Answer from the drawing. Dimensions are ordinates in mm from the lowest x, y and z of the part. A direction names the side the tool comes from. Coordinates: 2 decimals unless noted, no trailing zeros. Loops run counter-clockwise (first coordinate to the right, second up) from the corner with the lowest first, then second, coordinate; pieces in that order, holes last.
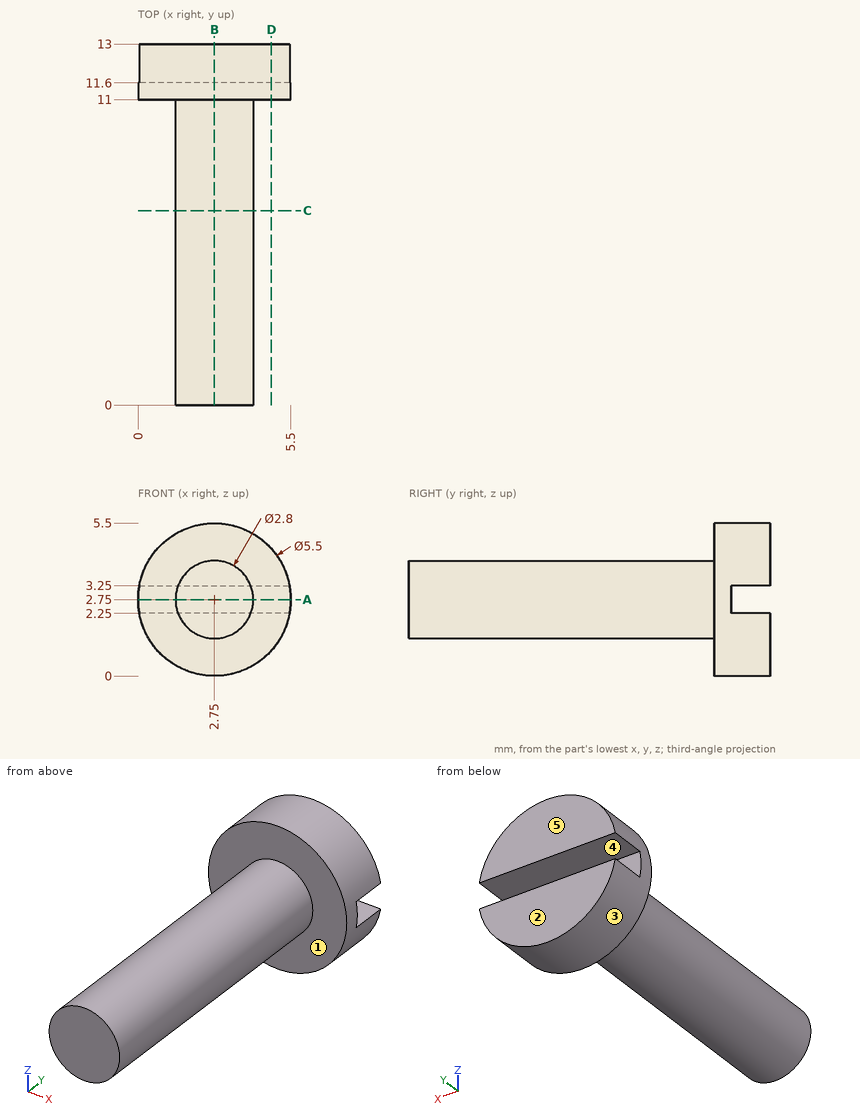
Item 1: A cutting plane is placed at B-B on x = 2.75. Determine the outline of the cut face in (y, z).
Numbers:
outline: (0, 1.35) - (11, 1.35) - (11, 0) - (13, 0) - (13, 2.25) - (11.6, 2.25) - (11.6, 3.25) - (13, 3.25) - (13, 5.5) - (11, 5.5) - (11, 4.15) - (0, 4.15) - close
Item 2: Which of the six approach directions +Z, -Z, +X, -X, +Y, -Y give full straight-line access (tool end or side, diameter ignored) to the marked faces 1 and 2?
Numbers:
face 1: -Y
face 2: +Z, -Z, +X, -X, +Y
Item 3: A cutting plane is placed at D-D on x = 4.8. Determine the outline of the cut face in (y, z), then the cut area to 3 significant figures.
Numbers:
outline: (11, 0.92) - (13, 0.92) - (13, 2.25) - (11.6, 2.25) - (11.6, 3.25) - (13, 3.25) - (13, 4.58) - (11, 4.58) - close
area: 5.93 mm2
Item 4: A cutting plane is placed at A-A on z = 2.75. Determine the outline of the cut face in (x, y), then the cut area to 3 significant figures.
Numbers:
outline: (0, 11) - (1.35, 11) - (1.35, 0) - (4.15, 0) - (4.15, 11) - (5.5, 11) - (5.5, 11.6) - (0, 11.6) - close
area: 34.1 mm2
Item 5: Given pin 1 (1.5 mm diameter, centred on x = 2.5, y = 2, fed in from -Z); pin 2 (2 mm diameter, centred on y = 8.5, z = 1, fed in from +X), each flat-ended and moving along its own axis, determine where each tip first touches the part or whether it passes through.
Numbers:
pin 1: stops at z = 1.35
pin 2: stops at x = 3.93
Item 6: Determine the mould class of the marked faces 3, 4 and 5 for opening direction Z: released by +Z, released by -Z, zero draft, split by the parting line, or undercut.
Numbers:
face 3: split by the parting line
face 4: undercut
face 5: zero draft
Item 7: A cutting plane is placed at C-C on y = 7. Determine the outline of the cut face in (x, z), then the cut area to 3 significant figures.
Numbers:
outline: circle Ø2.8 at (2.75, 2.75)
area: 6.16 mm2
Item 8: Find the intervals of material crossed by line 1 along Y through (x, z) = (0.4, 2.7); line 2 along Z through (x, y) = (2.75, 8.5); line 3 along Y through (x, z) = (2.65, 3.2), in increasing order.
Numbers:
line 1: y = 11 to 11.6
line 2: z = 1.35 to 4.15
line 3: y = 0 to 11.6
